from build123d import *

# Parameters (mm, degrees)
SKETCH1_W           = 27
SKETCH1_H           = 37.5
BOSS_EXTRUDE1_DEPTH = 23
BOSS_EXTRUDE2_DEPTH = 2.25
FILLET1_R           = 3
FILLET2_R           = 1


with BuildPart() as part:
    # Sketch1 → Boss-Extrude1 (new body)
    with BuildSketch(Plane(origin=(0, 0, 0), x_dir=(1, 0, 0), z_dir=(0, 1, 0))):
        Rectangle(SKETCH1_W, SKETCH1_H)
    extrude(amount=BOSS_EXTRUDE1_DEPTH)

    # Sketch2 → Boss-Extrude2 (add)
    with BuildSketch(Plane(origin=(0, 0, 0), x_dir=(1, 0, 0), z_dir=(0, 1, 0))):
        with BuildLine():
            Line((-1.75, -22.5), (-1.75, -25.75))
            Line((-1.75, -25.75), (-2.575, -25.75))
            ThreePointArc((-2.575, -25.75), (-3.635660172, -25.310660172), (-4.075, -24.25))
            Line((-4.075, -24.25), (-4.075, -20.25))
            ThreePointArc((-4.075, -20.25), (-4.514339828, -19.189339828), (-5.575, -18.75))
            Line((-5.575, -18.75), (5.575, -18.75))
            ThreePointArc((5.575, -18.75), (4.514339828, -19.189339828), (4.075, -20.25))
            Line((4.075, -20.25), (4.075, -24.25))
            ThreePointArc((4.075, -24.25), (3.635660172, -25.310660172), (2.575, -25.75))
            Line((2.575, -25.75), (1.75, -25.75))
            Line((1.75, -25.75), (1.75, -22.5))
            ThreePointArc((1.75, -22.5), (0, -20.75), (-1.75, -22.5))
        make_face()
        with BuildLine():
            Line((1.75, 22.5), (1.75, 25.75))
            Line((1.75, 25.75), (2.575, 25.75))
            ThreePointArc((2.575, 25.75), (3.635660172, 25.310660172), (4.075, 24.25))
            Line((4.075, 24.25), (4.075, 20.25))
            ThreePointArc((4.075, 20.25), (4.514339828, 19.189339828), (5.575, 18.75))
            Line((5.575, 18.75), (-5.575, 18.75))
            ThreePointArc((-5.575, 18.75), (-4.514339828, 19.189339828), (-4.075, 20.25))
            Line((-4.075, 20.25), (-4.075, 24.25))
            ThreePointArc((-4.075, 24.25), (-3.635660172, 25.310660172), (-2.575, 25.75))
            Line((-2.575, 25.75), (-1.75, 25.75))
            Line((-1.75, 25.75), (-1.75, 22.5))
            ThreePointArc((-1.75, 22.5), (0, 20.75), (1.75, 22.5))
        make_face()
    extrude(amount=BOSS_EXTRUDE2_DEPTH)

    # Fillet1
    fillet1_edges = [part.edges().sort_by_distance(p)[0] for p in [
        (13.5, 23, 0),
        (-13.5, 23, 0),
    ]]
    fillet(fillet1_edges, radius=FILLET1_R)

    # Fillet2
    fillet2_edges = [part.edges().sort_by_distance(p)[0] for p in [
        (0, 23, 18.75),
        (0, 23, -18.75),
        (-13.5, 10, -18.75),
        (13.5, 10, -18.75),
        (-12.621320344, 22.121320344, -18.75),
        (12.621320344, 22.121320344, -18.75),
        (13.5, 10, 18.75),
        (-13.5, 10, 18.75),
        (-12.621320344, 22.121320344, 18.75),
        (12.621320344, 22.121320344, 18.75),
    ]]
    fillet(fillet2_edges, radius=FILLET2_R)


solid = part.part
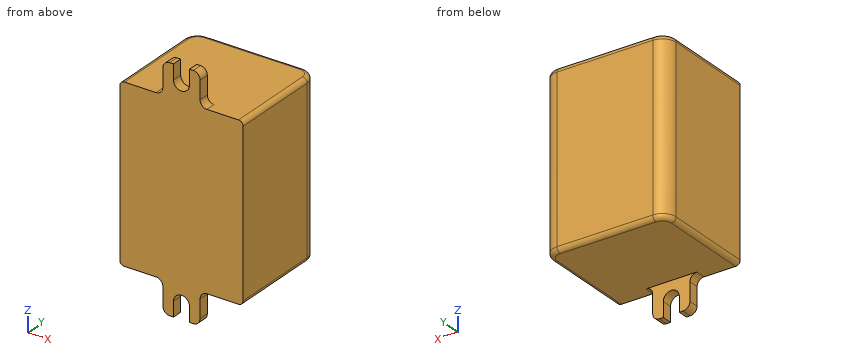
Here's how the part is built. I have some questions about the finished solid (model axes, mm). Coordinates: 2 decimals unless noted, no trailing zeros. Write each loop counter-clockwise with the first axis right and the second up, starting at its lowest first coordinate (ties: lowest second). Pieces come first, ordered by that corner, then holes. Notation, with made-up numbers: (49, -7) - (57, -7) arc R22 cw to (57, 8) - close; hole circle Ø11 at (9.25, 78). An arc over 180 degrees is marked (long way). Use one line per item in the form item = value.
1) Suppose I cut it at D-D, the plane x = 5. Write out the boundary of the cut face in (y, z), plus the area to 3 significant figures.
Solved:
outline = (0, -18.86) - (2.25, -18.86) - (2.25, -18.75) - (22, -18.75) arc R1 ccw to (23, -17.75) - (23, 17.75) arc R1 ccw to (22, 18.75) - (2.25, 18.75) - (2.25, 18.86) - (0, 18.86) - close
area = 863 mm2
2) Suppose I cut it at B-B, the plane y = 11.5. Write out the boundary of the cut face in (x, z), plus the area to 3 significant figures.
Solved:
outline = (-13.5, -17.75) arc R1 ccw to (-12.5, -18.75) - (12.5, -18.75) arc R1 ccw to (13.5, -17.75) - (13.5, 17.75) arc R1 ccw to (12.5, 18.75) - (-12.5, 18.75) arc R1 ccw to (-13.5, 17.75) - close
area = 1,010 mm2
3) Suppose I cut it at C-C, the plane x = -0.5. Write out the boundary of the cut face in (y, z).
Solved:
outline = (0, -20.82) - (2.25, -20.82) - (2.25, -18.75) - (22, -18.75) arc R1 ccw to (23, -17.75) - (23, 17.75) arc R1 ccw to (22, 18.75) - (2.25, 18.75) - (2.25, 20.82) - (0, 20.82) - close
4) Suppose I cut it at A-A, the plane z = -21.5. Write out the boundary of the cut face in (x, y) (3 decimals), plus the area to 3 significant figures.
Solved:
outline = (-4.075, 0) - (-1.436, 0) - (-1.436, 2.25) - (-4.075, 2.25) - close; (1.436, 0) - (4.075, 0) - (4.075, 2.25) - (1.436, 2.25) - close
area = 11.9 mm2
5) I need wall thicknesses on line 1 (Z direction, x = -5, y = 14); line 2 (Z direction, x = 0, y = 2); line 3 (Y direction, x = 0, z = -20). Which ranges of each line are inside material? Lowest first, please.
Solved:
line_1 = -18.75 to 18.75
line_2 = -20.75 to 20.75
line_3 = 0 to 2.25
6) I'm going to push flat-ended pins straight in: P1, Ø2.5, axis at y = 1.5, z = -24.5, coming from the +X side (3 decimals); P2, Ø5, axis at x = 8.5, y = 14.5, coming from the +Z side; P3, Ø4, axis at x = -3, y = 8, coming from the -Z side; P4, Ø12, axis at x = 3.5, z = 6, coming from the -Y side. Where does each tip first touch, or does it pass through?
Solved:
P1 = 4.075
P2 = 18.75
P3 = -18.75
P4 = 0
